Design review of the part built by this model. Coordinates are the model's own, in mm. Face numbers are marked on the shaded views. A direction names the side the tool comes from. Coordinates: 2 decimals unless noted, no trailing zeros. Loops run counter-clockwise (first coordinate to the right, second up) from the corner with the lowest first, then second, coordinate; pieces in that order, holes last. Notation, with made-up numbers: (-20, 66) - (31, 66) arc R37 ccw to (31, 103) - close; hole circle Ø9 at (37, 32.5). An arc over 180 degrees is marked (long way). Answer in a Markdown table with one row per item. Add a question column.
(1) For the marked faces 1 and 2, list the 3-axis set-ups (+Z, -Z, +X, -X, +Y, -Y) from which the entire face can be reached by the end or side of a thin tool; tool diameter is ignored.
(2) To check wall thickness, follow L1, parallel to X at y = 0.35, z = -12.7; L2, parallel to X at y = 0.15, z = -12; L3, parallel to Z at x = 10.5, y = 0.4. State the ranges of each line that lie inside material, in increasing order. Write a range as [from, to].
(3) We need section D-D, the plane z = -23.5. Write out the cut boundary in (x, y) (3 decimals).
(4) We need section A-A, the plane x = 11.43. Write out the cut boundary in (y, z) (3 decimals), plus the area to 3 significant figures.
(5) The part is to be moulded in two halves that separate along Z. For the marked faces 3, 4 and 5, say which applies: released by +Z, released by -Z, zero draft, split by the parting line, or undercut.
(6) We need section B-B, the plane y = 0.3. Write out the cut boundary in (x, z), plus the area to 3 significant figures.
(7) We need section C-C, the plane x = 6. Write out the cut boundary in (y, z) (3 decimals), plus the area to 3 significant figures.
from build123d import *

# Parameters (mm, degrees)
BOSS_EXTRUDE1_DEPTH = 22.86
SKETCH7_R           = 2.667
CUT_EXTRUDE1_DEPTH  = 22.86


with BuildPart() as part:
    # Sketch6 → Boss-Extrude1 (new body)
    with BuildSketch(Plane(origin=(0, 0, 0), x_dir=(0, 0, -1), z_dir=(1, 0, 0))):
        Polygon((0, 0), (25.4, 0), (25.4, 0.635), (22.225, 1.27), (19.05, 0.635), (15.875, 1.27), (12.7, 0.635), (9.525, 1.27), (6.35, 0.635), (3.175, 1.27), (0, 0.635), align=None)
    extrude(amount=BOSS_EXTRUDE1_DEPTH)

    # Sketch7 → Cut-Extrude1 (cut)
    with BuildSketch(Plane.XZ):
        with Locations(Location((11.43, -12.7, 0), (0, 0, 270))):
            Circle(SKETCH7_R)
    extrude(amount=-CUT_EXTRUDE1_DEPTH, mode=Mode.SUBTRACT)


solid = part.part
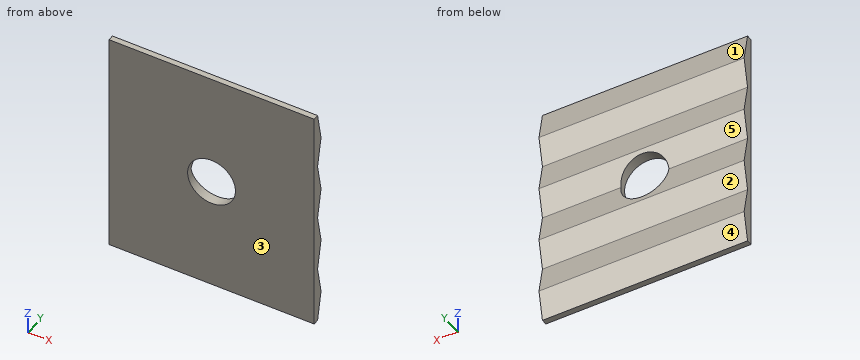
Responses:
| question | item | result |
|---|---|---|
| 1 | face 1 | +Z, +X, -X, +Y |
| 1 | face 2 | +X, -X, +Y |
| 2 | L1 | x = [0, 8.76], [14.1, 22.86] |
| 2 | L2 | x = [0, 8.86], [14, 22.86] |
| 2 | L3 | z = [-25.4, -15.2], [-10.2, 0] |
| 3 | outline | (0, 0) - (22.86, 0) - (22.86, 1.015) - (0, 1.015) - close |
| 4 | outline | (0, -25.4) - (0.635, -25.4) - (1.27, -22.225) - (0.635, -19.05) - (1.27, -15.875) - (1.168, -15.367) - (0, -15.367) - close; (0, -10.033) - (1.168, -10.033) - (1.27, -9.525) - (0.635, -6.35) - (1.27, -3.175) - (0.635, 0) - (0, 0) - close |
| 4 | area | 19.4 mm2 |
| 5 | face 3 | zero draft |
| 5 | face 4 | released by -Z |
| 5 | face 5 | undercut |
| 6 | outline | (0, -25.4) - (22.86, -25.4) - (22.86, 0) - (0, 0) - close; hole circle Ø5.33 at (11.43, -12.7) |
| 6 | area | 558 mm2 |
| 7 | outline | (0, -25.4) - (0.635, -25.4) - (1.27, -22.225) - (0.635, -19.05) - (1.27, -15.875) - (0.635, -12.7) - (1.27, -9.525) - (0.635, -6.35) - (1.27, -3.175) - (0.635, 0) - (0, 0) - close |
| 7 | area | 24.2 mm2 |
